from build123d import *

# Parameters (mm, degrees)
SKETCH1_R           = 3.67931812
SKETCH1_R_2         = 0.75
BOSS_EXTRUDE1_DEPTH = 1
SKETCH2_R           = 3.67931812
BOSS_EXTRUDE2_DEPTH = 5
SKETCH2_3_R         = 1.5
CUT_EXTRUDE1_DEPTH  = 0.5
SKETCH1_2_R         = 0.75
CUT_EXTRUDE2_DEPTH  = 19.333027078
SKETCH3_R           = 2.355
CUT_EXTRUDE3_DEPTH  = 2


with BuildPart() as part:
    # Sketch1 → Boss-Extrude1 (new body)
    # profile 1 of 2: a face of its own
    with BuildSketch(Plane(origin=(0, 0, 0), x_dir=(1, 0, 0), z_dir=(0, 1, 0))):
        Circle(SKETCH1_R)
        with Locations(Location((0, 0, 0), (0, 0, 270))):
            Circle(SKETCH1_R_2, mode=Mode.SUBTRACT)
    # profile 2 of 2: a face of its own
    with BuildSketch(Plane(origin=(0, 0, 0), x_dir=(1, 0, 0), z_dir=(0, 1, 0))):
        with BuildLine():
            ThreePointArc((2.49119588, 14.959626071), (0, 17.25), (-2.49119588, 14.959626071))
            Line((-2.49119588, 14.959626071), (-3.608885156, 1.677008569))
            ThreePointArc((-3.608885156, 1.677008569), (-3.66170212, 0.839243514), (-3.67931812, 4.9e-08))
            ThreePointArc((-3.67931812, 4.9e-08), (2.4e-08, 3.67931812), (3.67931812, 0))
            ThreePointArc((3.67931812, 0), (3.661702121, 0.83924349), (3.608885156, 1.677008569))
            Line((3.608885156, 1.677008569), (2.49119588, 14.959626071))
        make_face()
        with Locations(Location((0, 4.75, 0), (0, 0, 270))):
            Circle(SKETCH1_R_2, mode=Mode.SUBTRACT)
        with Locations(Location((0, 6.75, 0), (0, 0, 270))):
            Circle(SKETCH1_R_2, mode=Mode.SUBTRACT)
        with Locations(Location((0, 8.75, 0), (0, 0, 270))):
            Circle(SKETCH1_R_2, mode=Mode.SUBTRACT)
        with Locations(Location((0, 10.75, 0), (0, 0, 270))):
            Circle(SKETCH1_R_2, mode=Mode.SUBTRACT)
        with Locations(Location((0, 12.75, 0), (0, 0, 270))):
            Circle(SKETCH1_R_2, mode=Mode.SUBTRACT)
        with Locations(Location((0, 14.75, 0), (0, 0, 270))):
            Circle(SKETCH1_R_2, mode=Mode.SUBTRACT)
    extrude(amount=BOSS_EXTRUDE1_DEPTH)

    # Sketch2 → Boss-Extrude2 (add)
    with BuildSketch(Plane.XZ):
        with Locations(Location((0, 0, 0), (0, 0, 270))):
            Circle(SKETCH2_R)
    extrude(amount=-BOSS_EXTRUDE2_DEPTH)

    # Sketch2_3 → Cut-Extrude1 (cut)
    with BuildSketch(Plane.XZ):
        with Locations(Location((0, 0, 0), (0, 0, 270))):
            Circle(SKETCH2_3_R)
    extrude(amount=-CUT_EXTRUDE1_DEPTH, mode=Mode.SUBTRACT)

    # Sketch1_2 → Cut-Extrude2 (cut, through all)
    with BuildSketch(Plane(origin=(0, 0, 0), x_dir=(1, 0, 0), z_dir=(0, 1, 0))):
        with Locations(Location((0, 0, 0), (0, 0, 90))):
            Circle(SKETCH1_2_R)
    extrude(amount=CUT_EXTRUDE2_DEPTH, mode=Mode.SUBTRACT)

    # Sketch3 → Cut-Extrude3 (cut)
    with BuildSketch(Plane(origin=(0, 5, 0), x_dir=(1, 0, 0), z_dir=(0, 1, 0))):
        with Locations(Location((0, 0, 0), (0, 0, 270))):
            Circle(SKETCH3_R)
    extrude(amount=-CUT_EXTRUDE3_DEPTH, mode=Mode.SUBTRACT)


solid = part.part
Work out the finished part from the listing and answer in its coordinate system (mm). A direction names the side the tool comes from. Round coordinates to 2 decimals unless told otherwise and drop trailing zeros. Write each loop counter-clockwise with the first axis right and the second up, starting at its lowest first coordinate (ties: lowest second). Pieces come first, ordered by that corner, then holes. Notation, with made-up numbers: M -40,5.25 L -16,5.25 A24 ccw -16,22.25 Z; hole C 2.5,-37.75 d9. An arc over 180 degrees is marked long. Use a Markdown table: item, result.
1) The part is cut by section D-D on z = -8.5. Give the vertices of the cut face in (x, y).
Taken from the geometry:
| item | result |
|---|---|
| outline | M -3.03,0 L -0.71,0 L -0.71,1 L -3.03,1 Z; M 0.71,0 L 3.03,0 L 3.03,1 L 0.71,1 Z |
2) Determine the mould class of faces 4 (the face through (1, 3, -1)), 5 (the face through (-3.66, 0.49, -0.85)), 6 (the face through (1, 1, -9)) for opening direction X: pulls with the +X half, pulls with the -X half, needs draft (parallel to the pull), parting line crosses it, or undercut.
Taken from the geometry:
| item | result |
|---|---|
| face 4 | undercut |
| face 5 | pulls with the -X half |
| face 6 | needs draft |
3) The part is cut by section A-A on z = -12.75. Give the vertices of the cut face in (x, y).
Taken from the geometry:
| item | result |
|---|---|
| outline | M -2.68,0 L -0.75,0 L -0.75,1 L -2.68,1 Z; M 0.75,0 L 2.68,0 L 2.68,1 L 0.75,1 Z |
4) Flat-ended cylindrical pins translate along their axes: pin 1 (2.5 mm diameter, centred on x = 0, z = -6.75, fed in from +Y); pin 2 (1.5 mm diameter, centred on x = 0.5, z = 0.5, fed in from -Y); pin 3 (1 mm diameter, centred on x = -2, z = 0.5, fed in from -Y); pin 4 (1.2 mm diameter, centred on x = 0, z = -14.75, fed in from -Y). Find the tip coordinate at first contact, or state that the pin passes through.
Taken from the geometry:
| item | result |
|---|---|
| pin 1 | stops at y = 1 |
| pin 2 | stops at y = 0.5 |
| pin 3 | stops at y = 0 |
| pin 4 | passes through |
5) Consider line 1 (X direction, y = 2.4, z = 0); line 2 (Z direction, x = -1.75, y = 3.75); line 3 (Z direction, x = -1, y = 4.4). Determine where each line is inside the solid, lowest interval first. Write a range as [from, to].
Taken from the geometry:
| item | result |
|---|---|
| line 1 | x = [-3.68, -0.75], [0.75, 3.68] |
| line 2 | z = [-3.24, -1.58], [1.58, 3.24] |
| line 3 | z = [-3.54, -2.13], [2.13, 3.54] |
6) Which of the six approach directions +Z, -Z, +X, -X, +Y, -Y give full straight-line access (tool end or side, diameter ignored) to faces 1 (the face through (1, 0.5, 0)), 2 (the face through (-3.042, 0.493, -8.411)), 3 (the face through (-2.3, 4, -0.5))?
Taken from the geometry:
| item | result |
|---|---|
| face 1 | -Y |
| face 2 | -Z, -X, +Y, -Y |
| face 3 | +Y |
7) The part is cut by section C-C on x = 0. State how many separate pieces and enclosed holes the cut face has, plus the area to 3 significant figures.
Taken from the geometry:
| item | result |
|---|---|
| separate pieces | 8 |
| enclosed holes | 0 |
| area | 26.7 mm2 |
8) The part is cut by section B-B on y = 1.85. Give the vertices of the cut face in (x, z).
Taken from the geometry:
| item | result |
|---|---|
| outline | C 0,0 d7.36; hole C 0,0 d1.5 |
